Autodesk Inventor part; units mm, degrees
ref_plane "YZ Plane" through (0, 0, 0) normal (1, 0, 0) x (0, 1, 0)
ref_plane "XZ Plane" through (0, 0, 0) normal (0, 1, 0) x (-1, 0, 0)
ref_plane "XY Plane" through (0, 0, 0) normal (0, 0, 1) x (1, 0, 0)
sketch "スケッチ1" plane through (0, 0, 0) normal (0, 0, 1) x (1, 0, 0)
  circle A0 centre (0, 0) radius 10.25
  dimension "d0" = 20.5
extrude "押し出し1" add sketch "スケッチ1" along normal blind 2
sketch "スケッチ2" plane through (0, 0, 0) normal (0, 0, -1) x (-1, 0, 0)
  circle A0 centre (0, 0) radius 4.1
  dimension "d3" = 8.2
extrude "押し出し2" add sketch "スケッチ2" along normal blind 4.5
sketch "スケッチ3" plane through (0, 0, -4.5) normal (0, 0, -1) x (-1, 0, 0)
  point P0 (0, 0)
  point P1 (0, 0)
hole "穴1" at (0, 0, -4.5) direction (0, 0, 1) diameter 3 end through all counterbore diameter 6 counterbore depth 4
sketch "スケッチ4" plane through (0, 0, 2) normal (0, 0, 1) x (1, 0, 0)
  point P0 (0, 0)
  point P1 (7.5, 0)
  point P2 (0, 7.5)
  point P3 (-7.5, 0)
  point P4 (0, -7.5)
  dimension "d13" = 7.5
  dimension "d16" = 360
hole "穴2" at (7.5, 0, 2) at (0, 7.5, 2) at (-7.5, 0, 2) at (0, -7.5, 2) direction (0, 0, -1) diameter 3 end through all
sketch "スケッチ5" plane through (0, 0, 2) normal (0, 0, 1) x (1, 0, 0)
  circle A0 centre (7.5, 0) radius 1.5
  point P0 (0, 0)
  point P1 (7.5, 3.5)
  point P2 (7.5, -3.5)
  point P3 (-3.5, 7.5)
  point P4 (3.5, 7.5)
  point P5 (-7.5, -3.5)
  point P6 (-7.5, 3.5)
  point P7 (3.5, -7.5)
  point P8 (-3.5, -7.5)
  dimension "d25" = 3.5
  dimension "d26" = 3.5
  dimension "d29" = 360
hole "穴3" at (7.5, 3.5, 2) at (7.5, -3.5, 2) at (-3.5, 7.5, 2) at (3.5, 7.5, 2) at (-7.5, -3.5, 2) at (-7.5, 3.5, 2) at (3.5, -7.5, 2) at (-3.5, -7.5, 2) direction (0, 0, -1) diameter 1 end through all
properties part number "ServoHorn_Circle" material "ABS プラスチック"
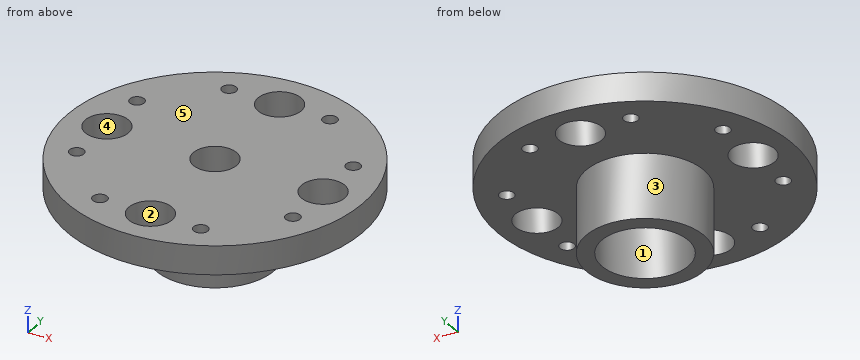
Work out the finished part from the listing and answer in its coordinate system (mm). Face numbers are marked on the shaded views. A direction names the side the tool comes from. Coordinates: 2 decimals unless noted, no trailing zeros. Loops run counter-clockwise (first coordinate to the right, second up) from the corner with the lowest first, then second, coordinate; pieces in that order, holes last. Notation, with made-up numbers: M 19,15 L 65,15 A19 cw 65,49 Z; hole C 10,57.25 d9. An arc over 180 degrees is marked long. Answer in a Markdown table with one row per item. Add a question column.
1. Find section D-D, the plane x = -8.5. Write down the section's boundary in (y, z), then the cut area to 3 significant figures.
2. Find section A-A, the plane x = 0. Write down the section's boundary in (y, z).
3. Flat-ended cylindrical pins translate along their axes: P1, Ø2.5, axis at x = 0, y = 0, coming from the +Z side; P2, Ø4, axis at x = -7.5, y = 0, coming from the -Z side; P3, Ø3.5, axis at x = 0, y = 0, coming from the -Z side; P4, Ø10, axis at x = -1, y = 5.5, coming from the -Z side. Find the tip coordinate at first contact, or state that the pin passes through.
4. Find section C-C, the plane z = 0.25. State how many separate pieces and enclosed holes the cut face has, then the cut area to 3 significant figures.
5. The mould has two halves that part along Y. Classify the marked faces 3, 4 and 5: pulls with the +Y half, pulls with the -Y half, needs draft (parallel to the pull), parting line crosses it, or undercut.
6. A tool of negligible diameter and unlimited length cuts with its end or side. For the marked faces 1 and 2, from which of +Z, -Z, +X, -X, +Y, -Y can it reach the whole face along a straight path? Write none if from no direction.
7. Consider L1, parallel to Y at x = 0, z = 0.6; L2, parallel to Y at x = 7.5, z = 1; L3, parallel to Y at x = -3.5, z = 1.15. Determine where each line is inside the solid, lowest interval first.
Reported:
| question | item | result |
|---|---|---|
| 1 | outline | M -5.73,0 L -1.12,0 L -1.12,2 L -5.73,2 Z; M 1.12,0 L 5.73,0 L 5.73,2 L 1.12,2 Z |
| 1 | area | 18.4 mm^2 |
| 2 | outline | M -10.25,0 L -9,0 L -9,2 L -10.25,2 Z; M -6,0 L -4.1,0 L -4.1,-4.5 L -3,-4.5 L -3,-0.5 L -1.5,-0.5 L -1.5,2 L -6,2 Z; M 1.5,-0.5 L 3,-0.5 L 3,-4.5 L 4.1,-4.5 L 4.1,0 L 6,0 L 6,2 L 1.5,2 Z; M 9,0 L 10.25,0 L 10.25,2 L 9,2 Z |
| 3 | P1 | passes through |
| 3 | P2 | stops at z = 0 |
| 3 | P3 | stops at z = -0.5 |
| 3 | P4 | stops at z = -4.5 |
| 4 | separate pieces | 1 |
| 4 | enclosed holes | 13 |
| 4 | area | 288 mm^2 |
| 5 | face 3 | parting line crosses it |
| 5 | face 4 | undercut |
| 5 | face 5 | needs draft |
| 6 | face 1 | -Z |
| 6 | face 2 | +Z, -Z |
| 7 | L1 | y = -10.25 to -9, -6 to -1.5, 1.5 to 6, 9 to 10.25 |
| 7 | L2 | y = -6.99 to -4, -3 to -1.5, 1.5 to 3, 4 to 6.99 |
| 7 | L3 | y = -9.63 to -8, -7 to 7, 8 to 9.63 |
